Here's the drawing with two shaded views (mm, measured from the low corner). I have some questions. A direction names the side the tool comes from. Round coordinates to 2 decimals unless told otherwise and drop trailing zeros. Order: outer loops, then holes, each group sorted by start corner. A loop starts at its lowest first (then second) coordinate and runs counter-clockwise, first axis right, second up. Notation, with made-up numbers: (-2.5, 81) -> (49.5, 81) arc R21 ccw to (49.5, 87) -> close; hole circle Ø1 at (52.5, 37.25). An arc over 180 degrees is marked (long way). Use a Markdown table: item, result. Add a question column.
Q1. I need wall thicknesses on line 1 along Z through (x, y) = (33.5, 11.75); line 2 along Z through (x, y) = (6, 14.5); line 3 along X through (y, z) = (19, 20). Which ranges of each line are inside material? Lowest first, please. Write a range as [from, to].
Q2. We'd pull the mould along X, two halves only. Please class the marked faces 6, 7, 8 and 9: +X half, -X half, draft (parallel to the pull), parting line (faces both ways), or undercut.
Q3. I'm going to push flat-ended pins straight in: pin 1 Ø10 at (x, y) = (29.16, 8.2) entering from -Z; pin 2 Ø2 at (y, z) = (3, 3.5) entering from +X; pin 3 Ø4 at (x, z) = (8.5, 5) entering from -Y; pin 4 Ø4 at (x, y) = (16, 19.5) entering from +Z. Where does each tip first touch, or does it pass through?
Q4. If we section it at A-A on x = 13.5: List the corners of the cut face in (y, z) for me.
Q5. If we section it at D-D on x = 22.5: List the corners of the cut face in (y, z) for me.
Q6. For the marked faces 1, 2, 3, 4 and 5, which set-ups out of +Z, -Z, +X, -X, +Y, -Y let a thin tool reach every point of the face, with its end or its side?
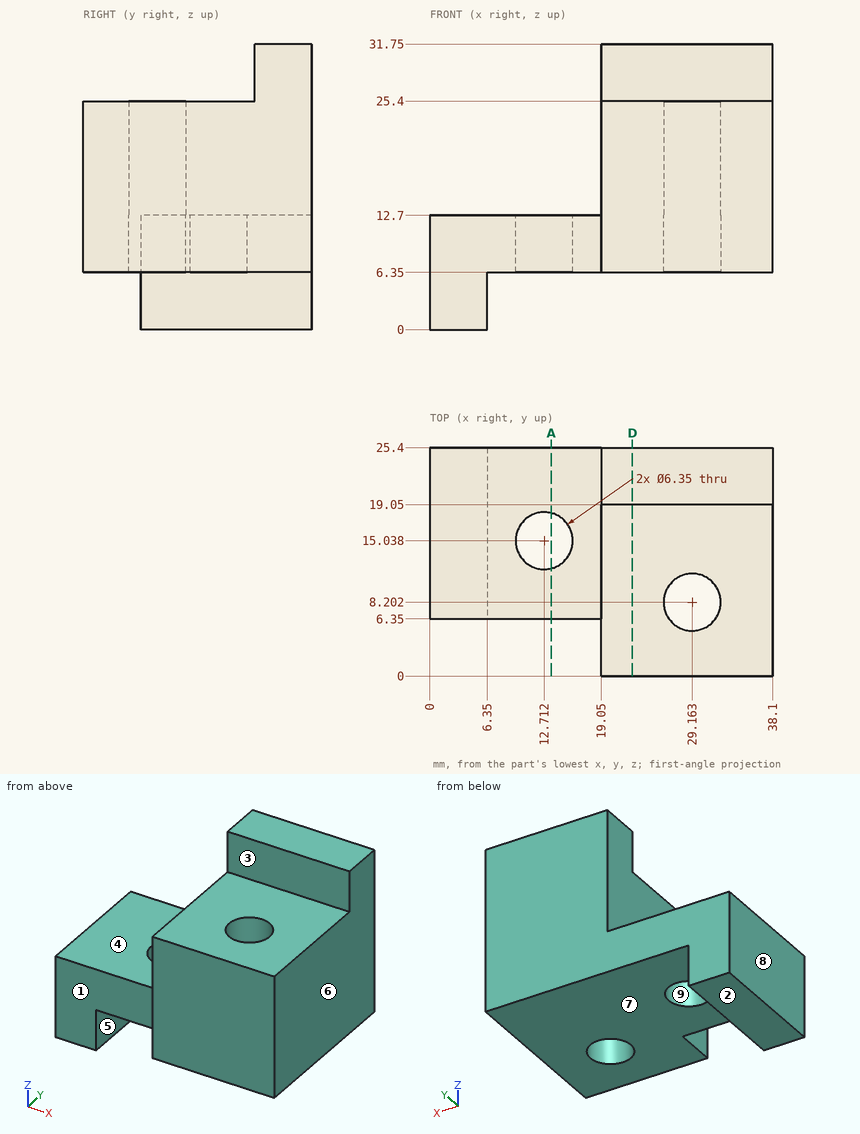
Answer below:
| question | item | result |
|---|---|---|
| 1 | line 1 | [6.35, 25.4] |
| 1 | line 2 | [0, 12.7] |
| 1 | line 3 | [19.05, 38.1] |
| 2 | face 6 | +X half |
| 2 | face 7 | draft |
| 2 | face 8 | -X half |
| 2 | face 9 | undercut |
| 3 | pin 1 | z = 6.35 |
| 3 | pin 2 | through |
| 3 | pin 3 | y = 6.35 |
| 3 | pin 4 | z = 12.7 |
| 4 | outline | (6.35, 6.35) -> (11.96, 6.35) -> (11.96, 12.7) -> (6.35, 12.7) -> close; (18.11, 6.35) -> (25.4, 6.35) -> (25.4, 12.7) -> (18.11, 12.7) -> close |
| 5 | outline | (0, 6.35) -> (25.4, 6.35) -> (25.4, 31.75) -> (19.05, 31.75) -> (19.05, 25.4) -> (0, 25.4) -> close |
| 6 | face 1 | +Z, -Z, -X, -Y |
| 6 | face 2 | -Z, +X, -X, +Y, -Y |
| 6 | face 3 | +Z, +X, -X, -Y |
| 6 | face 4 | +Z, -X, +Y, -Y |
| 6 | face 5 | -Z, +X, +Y, -Y |
